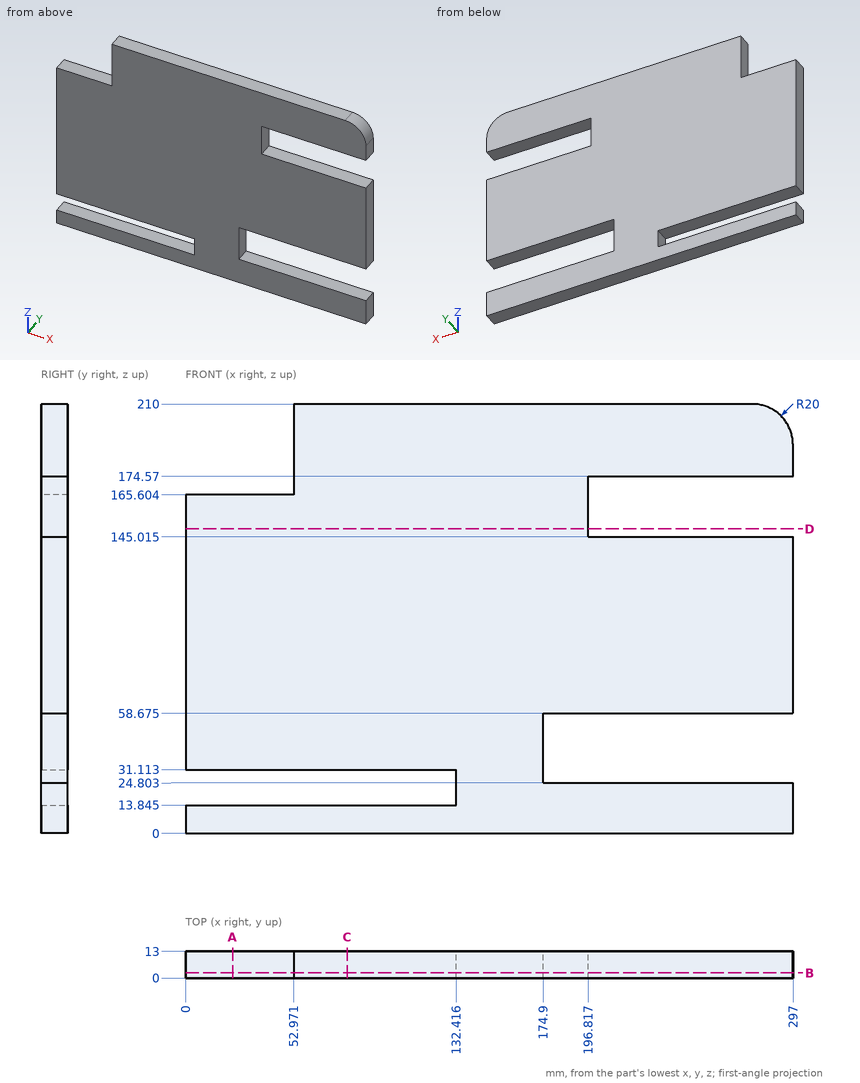
Answer from the drawing. Dimensions are ordinates in mm from the lowest x, y and z of the part. Give positions to 0.01 mm unless a question says otherwise; leave off trailing zeros. Loops run counter-clockwise (first coordinate to the right, second up) from the corner with the lowest first, then second, coordinate; pieces in that order, holes last. Notation, with made-up numbers: (54, 80) - (95, 80) arc R22 ccw to (95, 102) - close; hole circle Ø3 at (84, 16). An arc over 180 degrees is marked (long way). Answer as a JSON object with one key per item and string values.
1. Find the intervals of material crossed by L1, parallel to Z at x = 232.5, y = 5 (1 decimal); L2, parallel to Z at x = 100, y = 4.25 (1 decimal); L3, parallel to Z at x = 285, y = 10.25 (1 decimal), in increasing order. Write a range as [from, to].
Determined:
{"L1": "[0, 24.8], [58.7, 145], [174.6, 210]", "L2": "[0, 13.8], [31.1, 210]", "L3": "[0, 24.8], [58.7, 145], [174.6, 208.3]"}
2. A cutting plane is placed at C-C (x = 79). Write down the section's boundary in (y, z) (1 decimal).
Determined:
{"outline": "(0, 0) - (13, 0) - (13, 13.8) - (0, 13.8) - close; (0, 31.1) - (13, 31.1) - (13, 210) - (0, 210) - close"}
3. A cutting plane is placed at D-D (z = 149). Write down the section's boundary in (x, y), then the cut area to 3 significant figures.
Determined:
{"outline": "(0, 0) - (196.82, 0) - (196.82, 13) - (0, 13) - close", "area": "2,560 mm²"}
4. A cutting plane is placed at B-B (y = 2.5). Write down the section's boundary in (x, z) (1 decimal), then the cut area to 4 significant figures.
Determined:
{"outline": "(0, 0) - (297, 0) - (297, 24.8) - (174.9, 24.8) - (174.9, 58.7) - (297, 58.7) - (297, 145) - (196.8, 145) - (196.8, 174.6) - (297, 174.6) - (297, 190) arc R20 ccw to (277, 210) - (53, 210) - (53, 165.6) - (0, 165.6) - (0, 31.1) - (132.4, 31.1) - (132.4, 13.8) - (0, 13.8) - close", "area": "50,550 mm²"}
5. A flat-ended cylindrical pin translates along its axis: pin 1 Ø4 at (y, z) = (5.5, 192) entering from -X. Find the tip coordinate at first contact, or state that the pin passes through.
Determined:
{"pin 1": "x = 52.97"}
6. A cutting plane is placed at A-A (x = 23). Write down the section's boundary in (y, z) (1 decimal), then the cut area to 3 significant figures.
Determined:
{"outline": "(0, 0) - (13, 0) - (13, 13.8) - (0, 13.8) - close; (0, 31.1) - (13, 31.1) - (13, 165.6) - (0, 165.6) - close", "area": "1,930 mm²"}
